from build123d import *

# Parameters (mm, degrees)
SKETCH2_R           = 3
BOSS_EXTRUDE1_DEPTH = 1
FILLET1_R           = 1


with BuildPart() as part:
    # Sketch2 → Boss-Extrude1 (new body)
    with BuildSketch(Plane(origin=(0, 0, 0), x_dir=(1, 0, 0), z_dir=(0, 1, 0))):
        Polygon((0, 24), (5, 24), (5, 29), (24, 29), (24, 24), (29, 24), (29, 5), (24, 5), (24, 0), (5, 0), (5, 5), (0, 5), align=None)
        with Locations(Location((14.5, 14.5, 0), (0, 0, 270))):
            Circle(SKETCH2_R, mode=Mode.SUBTRACT)
    extrude(amount=BOSS_EXTRUDE1_DEPTH)

    # Fillet1
    fillet1_edges = [part.edges().sort_by_distance(p)[0] for p in [
        (5, 0.5, -24),
        (24, 0.5, -24),
        (24, 0.5, -5),
        (5, 0.5, -5),
    ]]
    fillet(fillet1_edges, radius=FILLET1_R)


solid = part.part
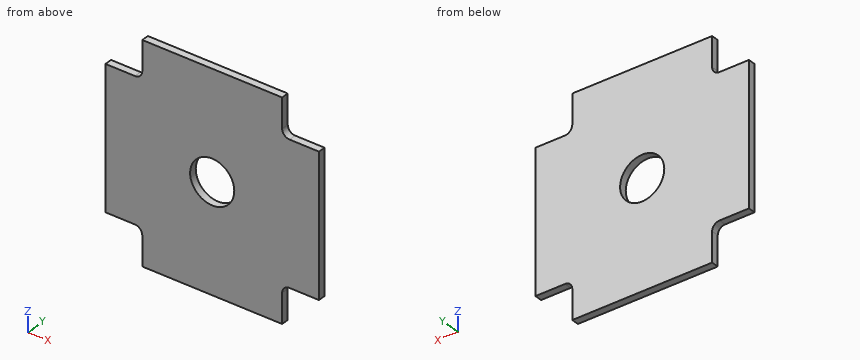
Geometry: final body of the model. Coordinates: model frame, mm. Give positions to 0.01 mm unless a question says otherwise; leave off trailing zeros. Loops run counter-clockwise (first coordinate to the right, second up) from the corner with the lowest first, then second, coordinate; pieces in that order, holes last. Notation, with made-up numbers: (-8.75, -37.5) -> (33.25, -37.5) arc R23 ccw to (33.25, -6.5) -> close; hole circle Ø2 at (-23.75, -4). An arc over 180 degrees is marked (long way). Put each result on its own line as item: value.
1. Cut plane D-D (x = 26). Return the cut outline in (y, z).
Taken from the geometry:
outline: (0, -24) -> (1, -24) -> (1, -5) -> (0, -5) -> close
2. Cut plane B-B (z = -14.5). Return the cut outline in (x, y).
Taken from the geometry:
outline: (0, 0) -> (11.5, 0) -> (11.5, 1) -> (0, 1) -> close; (17.5, 0) -> (29, 0) -> (29, 1) -> (17.5, 1) -> close
3. Cut plane A-A (x = 14.5). Return the cut outline in (y, z).
Taken from the geometry:
outline: (0, -29) -> (1, -29) -> (1, -17.5) -> (0, -17.5) -> close; (0, -11.5) -> (1, -11.5) -> (1, 0) -> (0, 0) -> close
4. Pin query (flat end, axial travel): P1, Ø3.5, axis at x = 14.5, z = -14.5, coming from the -Y side; P2, Ø2, axis at x = 4, z = -19, coming from the -Y side; P3, Ø0.5, axis at x = 28, y = 0.5, coming from the +Z side; P4, Ø0.5, axis at y = 0.5, z = -28, coming from the +X side. Return the tip coordinate at first contact, or that it passes through.
Taken from the geometry:
P1: passes through
P2: stops at y = 0
P3: stops at z = -5
P4: stops at x = 24
5. Cut plane C-C (y = 0.45). Return the cut outline in (x, z).
Taken from the geometry:
outline: (0, -24) -> (4, -24) arc R1 cw to (5, -25) -> (5, -29) -> (24, -29) -> (24, -25) arc R1 cw to (25, -24) -> (29, -24) -> (29, -5) -> (25, -5) arc R1 cw to (24, -4) -> (24, 0) -> (5, 0) -> (5, -4) arc R1 cw to (4, -5) -> (0, -5) -> close; hole circle Ø6 at (14.5, -14.5)
6. Ray query, line 1 along X through (y, z) = (0.65, -14.5); line 2 along Z through (x, y) = (27.25, 0.5); line 3 along Z through (x, y) = (17, 0.2). Return the intervals inside material, ascending. Write a range as [from, to].
Taken from the geometry:
line 1: x = [0, 11.5], [17.5, 29]
line 2: z = [-24, -5]
line 3: z = [-29, -16.16], [-12.84, 0]
